```python
from build123d import *

# Parameters (mm, degrees)
F0_R     = 39.780695
F0_R_2   = 31
F1_DEPTH = 88.9
F2_DEPTH = 2.54
F3_R     = 5.08


with BuildPart() as f1:
    # F0 (on Top) → F1 (new body)
    with BuildSketch(Plane.XY):
        Circle(F0_R)
        Circle(F0_R_2, mode=Mode.SUBTRACT)
    extrude(amount=F1_DEPTH)

    # F0 (on Top) → F2 (join)
    with BuildSketch(Plane.XY):
        Circle(F0_R_2)
    extrude(amount=F2_DEPTH)

    # F3
    f3_edges = [f1.edges().sort_by_distance(p)[0] for p in [
        (-31, 0, 88.9),
    ]]
    fillet(f3_edges, radius=F3_R)


solid = f1.part
```
Read the model definition and answer for the solid it produces. Units are mm, in the model's axes. A direction names the side the tool comes from. Coordinates: 2 decimals unless noted, no trailing zeros. Loops run counter-clockwise (first coordinate to the right, second up) from the corner with the lowest first, then second, coordinate; pieces in that order, holes last. Notation, with made-up numbers: (-29.5, 55.25) -> (-14.5, 55.25) arc R8 cw to (-14.5, 62.25) -> close; hole circle Ø11 at (14.25, 10). An arc over 180 degrees is marked (long way). Return JSON: item names as keys, results as strings.
Item 1: Find the intervals of material crossed by probe 1 along Y at (x, z) = (0, 55); probe 2 along Z at (x, y) = (-17.5, 6); probe 3 along X at (y, z) = (27, 77), in increasing order.
Answers:
{"probe 1": "y = -39.78 to -31, 31 to 39.78", "probe 2": "z = 0 to 2.54", "probe 3": "x = -29.21 to -15.23, 15.23 to 29.21"}
Item 2: Find section C-C (z = 60.5). Determine the outline of the cut face in (x, y).
Answers:
{"outline": "circle Ø79.56 at (0, 0); hole circle Ø62 at (0, 0)"}
Item 3: For faces 1 (the flat face through (0, 0, 2.54)), 2 (the flat face through (8.7, -35.2, 88.9)), determine the directions among +Z, -Z, +X, -X, +Y, -Y from which every point of the face is accessible in a straight line to the end or side of a thin tool.
Answers:
{"face 1": "+Z", "face 2": "+Z, +X, -X, +Y, -Y"}
Item 4: Find section A-A (x = 0). Determine the outline of the cut face in (y, z), plus the area to 3 significant figures.
Answers:
{"outline": "(-39.78, 0) -> (39.78, 0) -> (39.78, 88.9) -> (36.08, 88.9) arc R5.08 ccw to (31, 83.82) -> (31, 2.54) -> (-31, 2.54) -> (-31, 83.82) arc R5.08 ccw to (-36.08, 88.9) -> (-39.78, 88.9) -> close", "area": "1,710 mm2"}
Item 5: Flat-ended cylindrical pins translate along their axes: P1, Ø5, axis at x = -19, z = 12, coming from the +Y side; P2, Ø5, axis at y = 23.5, z = 48.5, coming from the -X side; P3, Ø10, axis at x = -5.5, z = 72, coming from the -Y side; P4, Ø6, axis at x = -7.5, y = -14.5, coming from the -Z side. Find the tip coordinate at first contact, or state that the pin passes through.
Answers:
{"P1": "stops at y = 36.2", "P2": "stops at x = -33.79", "P3": "stops at y = -39.78", "P4": "stops at z = 0"}
Item 6: For a pull along X with two mould halves and no side action, classify faces 3 (the flat face through (-1, 1, 0)), 4 (the cylindrical face through (-4.036, 30.736, 42.611)), 5 (the cylindrical face through (-8.624, -38.835, 43.828)) as +X half, -X half, draft (parallel to the pull), parting line (faces both ways), or undercut.
Answers:
{"face 3": "draft", "face 4": "undercut", "face 5": "parting line"}
